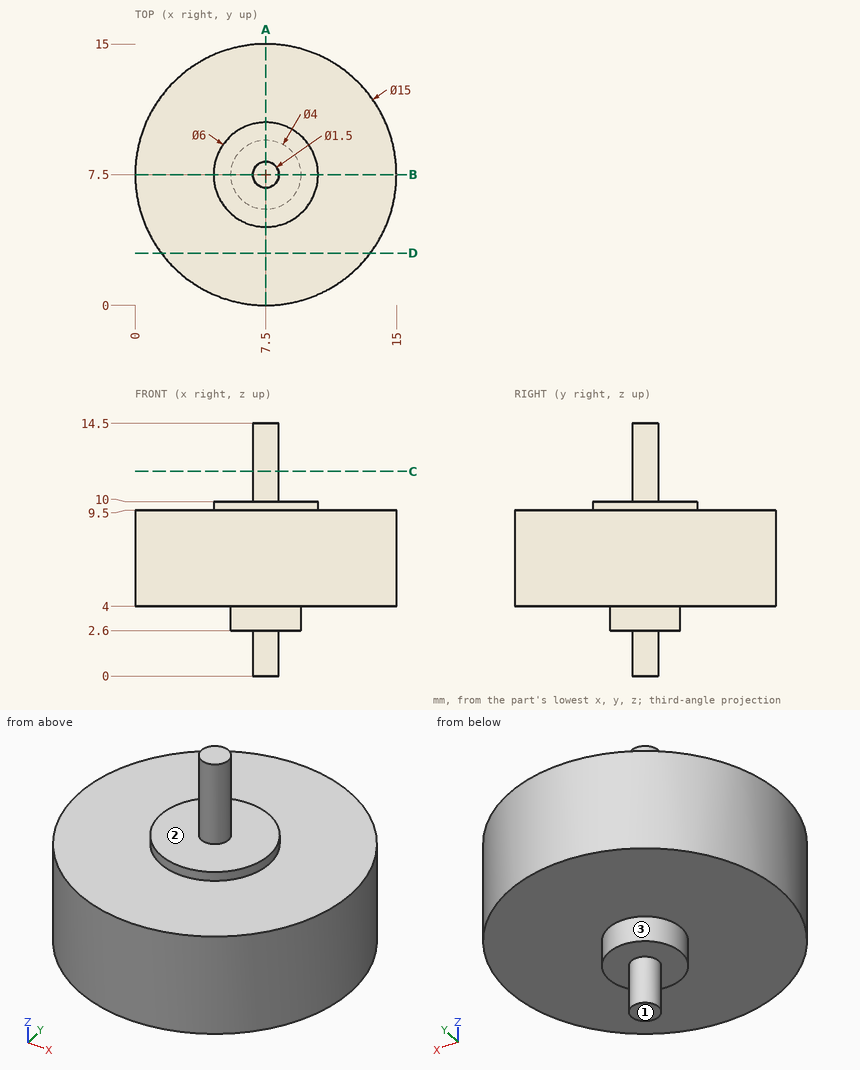
The figure shows three views and two pictorial views of one solid part (mm, origin at its lowest corner). Answer the questions. A direction names the side the tool comes from. Coordinates: 2 decimals unless noted, no trailing zeros. Write each loop counter-clockwise with the first axis right and the second up, starting at its lowest first coordinate (ties: lowest second). Pieces come first, ordered by that corner, then holes. Notation, with made-up numbers: (-10.5, -26.75) -> (25.5, -26.75) arc R19 cw to (25.5, -16.75) -> close; hole circle Ø1 at (-5.75, -32). An arc over 180 degrees is marked (long way). Return JSON: item names as keys, results as strings.
(1) The part is cut by section D-D on y = 3. Give the vertices of the cut face in (x, z).
Answers below:
{"outline": "(1.5, 4) -> (13.5, 4) -> (13.5, 9.5) -> (1.5, 9.5) -> close"}
(2) Consider line 1 along Z through (x, y) = (6, 10); line 2 along Z through (x, y) = (8.5, 8.75); line 3 along Y through (x, z) = (7.25, 1.5). Determine where each line is inside the solid, lowest interval first. Write a range as from..to.
Answers below:
{"line 1": "4..10", "line 2": "2.6..10", "line 3": "6.79..8.21"}
(3) Each of these flat-tipped pins is pushed along its axis until it touches: P1, Ø3, axis at x = 3.5, z = 4.5, coming from the +Y side; P2, Ø1.5, axis at x = 2.5, z = 12, coming from the +Y side; P3, Ø4, axis at x = 13, y = 3.5, coming from the -Z side. Where does it stop, or does it pass through?
Answers below:
{"P1": "y = 14.57", "P2": "through", "P3": "z = 4"}
(4) The part is cut by section A-A on x = 7.5. Give the vertices of the cut face in (y, z), then the cut area to 3 significant figures.
Answers below:
{"outline": "(0, 4) -> (5.5, 4) -> (5.5, 2.6) -> (6.75, 2.6) -> (6.75, 0) -> (8.25, 0) -> (8.25, 2.6) -> (9.5, 2.6) -> (9.5, 4) -> (15, 4) -> (15, 9.5) -> (10.5, 9.5) -> (10.5, 10) -> (8.25, 10) -> (8.25, 14.5) -> (6.75, 14.5) -> (6.75, 10) -> (4.5, 10) -> (4.5, 9.5) -> (0, 9.5) -> close", "area": "102 mm^2"}
(5) Which of the six approach directions +Z, -Z, +X, -X, +Y, -Y give full straight-line access (tool end or side, diameter ignored) to the marked faces 1, 2 and 3?
Answers below:
{"face 1": "-Z, +X, -X, +Y, -Y", "face 2": "+Z", "face 3": "-Z"}
(6) The part is cut by section C-C on z = 11.75. Give the vertices of the cut face in (x, y), then the cut area to 3 significant figures.
Answers below:
{"outline": "circle Ø1.5 at (7.5, 7.5)", "area": "1.77 mm^2"}
